```python
from build123d import *

# Parameters (mm, degrees)
CROQUIS1_W              = 37
CROQUIS1_H              = 38
SALIENTE_EXTRUIR1_DEPTH = 15
VACIADO1_T              = -4
CROQUIS2_W              = 6
CROQUIS2_H              = 8
CROQUIS2_R              = 1.5
SALIENTE_EXTRUIR2_DEPTH = 5
CROQUIS3_W              = 18
CROQUIS3_H              = 5
CORTAR_EXTRUIR1_DEPTH   = 5
CROQUIS4_R              = 1.5
SALIENTE_EXTRUIR3_DEPTH = 7
CROQUIS5_R              = 0.75
SALIENTE_EXTRUIR4_DEPTH = 7
CROQUIS7_R              = 1.5
CORTAR_EXTRUIR2_DEPTH   = 7


with BuildPart() as part:
    # Croquis1 → Saliente-Extruir1 (new body)
    with BuildSketch(Plane.XY):
        Rectangle(CROQUIS1_W, CROQUIS1_H)
    extrude(amount=SALIENTE_EXTRUIR1_DEPTH)

    # Vaciado1
    vaciado1_openings = [part.faces().sort_by_distance(p)[0] for p in [
        (0, 0, 15),
    ]]
    offset(amount=VACIADO1_T, openings=vaciado1_openings, kind=Kind.INTERSECTION)

    # Croquis2 → Saliente-Extruir2 (add)
    with BuildSketch(Plane.XY.offset(15)):
        with Locations((21.5, 0)):
            Rectangle(CROQUIS2_W, CROQUIS2_H)
        with Locations((21.5, 0)):
            Circle(CROQUIS2_R, mode=Mode.SUBTRACT)
    saliente_extruir2 = extrude(amount=-SALIENTE_EXTRUIR2_DEPTH)

    # Simetría1: Saliente-Extruir2 across plane
    add(saliente_extruir2.mirror(Plane(origin=(0, 0, 0), x_dir=(0, 0, 1), z_dir=(1, 0, 0))))

    # Croquis3 → Cortar-Extruir1 (cut)
    with BuildSketch(Plane.XZ.offset(19)):
        with Locations((0, 12.5)):
            Rectangle(CROQUIS3_W, CROQUIS3_H)
    extrude(amount=-CORTAR_EXTRUIR1_DEPTH, mode=Mode.SUBTRACT)

    # Croquis4 → Saliente-Extruir3 (add)
    with BuildSketch(Plane.XY.offset(4)):
        with Locations((-10.5, 10)):
            Circle(CROQUIS4_R)
        with Locations((10.5, 10)):
            Circle(CROQUIS4_R)
        with Locations((10.5, -3)):
            Circle(CROQUIS4_R)
        with Locations((-10.5, -3)):
            Circle(CROQUIS4_R)
    extrude(amount=SALIENTE_EXTRUIR3_DEPTH)

    # Croquis5 → Saliente-Extruir4 (add)
    with BuildSketch(Plane.XY.offset(11)):
        with Locations((-10.5, 10)):
            Circle(CROQUIS5_R)
        with Locations((10.5, 10)):
            Circle(CROQUIS5_R)
        with Locations((10.5, -3)):
            Circle(CROQUIS5_R)
        with Locations((-10.5, -3)):
            Circle(CROQUIS5_R)
    extrude(amount=SALIENTE_EXTRUIR4_DEPTH)

    # Croquis7 → Cortar-Extruir2 (cut)
    with BuildSketch(Plane.XY.offset(4)):
        with Locations((-6.5, 9)):
            Circle(CROQUIS7_R)
        with Locations((6.5, 9)):
            Circle(CROQUIS7_R)
        with Locations((6.5, -9)):
            Circle(CROQUIS7_R)
        with Locations((-6.5, -9)):
            Circle(CROQUIS7_R)
    extrude(amount=-CORTAR_EXTRUIR2_DEPTH, mode=Mode.SUBTRACT)


solid = part.part
```
The model under review builds one solid part; all positions refer to its coordinate system, in mm. A direction names the side the tool comes from. Coordinates: 2 decimals unless noted, no trailing zeros. Write each loop counter-clockwise with the first axis right and the second up, starting at its lowest first coordinate (ties: lowest second). Pieces come first, ordered by that corner, then holes. Notation, with made-up numbers: (58.25, 85.5) - (109.25, 85.5) arc R13 cw to (109.25, 95.5) - close; hole circle Ø11 at (35, 76.25). An arc over 180 degrees is marked (long way). Write item = value, one per line.
(1) For line 1 (Y direction, x = -5, z = 8); line 2 (Y direction, x = -6.5, z = 2.4); line 3 (X direction, y = 9.5, z = 2), list the stretches that pass through material, from the lowest coordinate up. Write a range as [from, to].
Result sheet:
line_1 = [-19, -15], [15, 19]
line_2 = [-19, -10.5], [-7.5, 7.5], [10.5, 19]
line_3 = [-18.5, -7.91], [-5.09, 5.09], [7.91, 18.5]
(2) Consider section B-B, the plane y = 0. Give the boundary of the cut face in (x, z), then the cut area to 3 significant figures.
Result sheet:
outline = (-24.5, 10) - (-23, 10) - (-23, 15) - (-24.5, 15) - close; (-20, 10) - (-18.5, 10) - (-18.5, 0) - (18.5, 0) - (18.5, 10) - (20, 10) - (20, 15) - (14.5, 15) - (14.5, 4) - (-14.5, 4) - (-14.5, 15) - (-20, 15) - close; (23, 10) - (24.5, 10) - (24.5, 15) - (23, 15) - close
area = 266 mm^2
(3) Mouldability with a two-part tool opening along Y and no side actions: class faces 6 (the face through (-9, -17, 12)), 7 (the face through (-21, -4, 13)), 8 (the face through (5.3, 8.1, 2)), 9 (the face through (5.3, -9.9, 2)) as pulls with the +Y half, pulls with the -Y half, needs draft (parallel to the pull), parting line crosses it, or undercut.
Result sheet:
face_6 = needs draft
face_7 = pulls with the -Y half
face_8 = undercut
face_9 = undercut
(4) Consider section A-A, the plane z = 12.5. Give the boundary of the cut face in (x, y).
Result sheet:
outline = (-24.5, -4) - (-18.5, -4) - (-18.5, -19) - (-9, -19) - (-9, -15) - (-14.5, -15) - (-14.5, 15) - (14.5, 15) - (14.5, -15) - (9, -15) - (9, -19) - (18.5, -19) - (18.5, -4) - (24.5, -4) - (24.5, 4) - (18.5, 4) - (18.5, 19) - (-18.5, 19) - (-18.5, 4) - (-24.5, 4) - close; circle Ø1.5 at (-10.5, -3); circle Ø1.5 at (-10.5, 10); circle Ø1.5 at (10.5, -3); circle Ø1.5 at (10.5, 10); hole circle Ø3 at (-21.5, 0); hole circle Ø3 at (21.5, 0)
(5) Machinability: for faces 1 (the face through (21, -4, 13)), 2 (the face through (11, -2, 11)), 3 (the face through (-20, 1, 10)), 4 (the face through (9, -17, 12)), 5 (the face through (23, 1, 10)), which of the approach directions +Z, -Z, +X, -X, +Y, -Y give a long, thin tool a straight path to every point of the face, cutting with its end or side? Answer none if there is none.
Result sheet:
face_1 = +Z, -Z, +X, -Y
face_2 = +Z
face_3 = -Z, -X, +Y, -Y
face_4 = +Z, -Y
face_5 = -Z, +X, +Y, -Y
(6) Consider section D-D, the plane y = -6.5. Give the boundary of the cut face in (x, z), then the cut area to 3 significant figures.
Result sheet:
outline = (-18.5, 0) - (18.5, 0) - (18.5, 15) - (14.5, 15) - (14.5, 4) - (-14.5, 4) - (-14.5, 15) - (-18.5, 15) - close
area = 236 mm^2
(7) Consider section C-C, the plane x = -10.5. Give the boundary of the cut face in (y, z).
Result sheet:
outline = (-19, 0) - (19, 0) - (19, 15) - (15, 15) - (15, 4) - (11.5, 4) - (11.5, 11) - (10.75, 11) - (10.75, 18) - (9.25, 18) - (9.25, 11) - (8.5, 11) - (8.5, 4) - (-1.5, 4) - (-1.5, 11) - (-2.25, 11) - (-2.25, 18) - (-3.75, 18) - (-3.75, 11) - (-4.5, 11) - (-4.5, 4) - (-15, 4) - (-15, 15) - (-19, 15) - close
(8) For P1, Ø4, axis at x = 22.5, z = 11.5, coming from the -Y side; P2, Ø8, axis at y = 9, z = 8, coming from the +X side; P3, Ø14.5, axis at x = -0.5, y = 3.5, coming from the +Z side; P4, Ø10, axis at x = 3.5, y = 6.5, coming from the -Z side, all flat-tipped, find the tip position at first contact; note any pin that passes through.
Result sheet:
P1 = -4
P2 = 18.5
P3 = 4
P4 = 0
